from build123d import *

# Parameters (mm, degrees)
ESBO_O1_R             = 5
EXTRUS_O1_DEPTH       = 29
ESBO_O1_3_R           = 6.35
EXTRUS_O2_DEPTH       = 3
ESBO_O2_R             = 1.75
CORTE_EXTRUS_O1_DEPTH = 7.5
CHANFRO1_SIZE         = 0.5


with BuildPart() as part:
    # Esbo_o1 → Extrus_o1 (new body)
    with BuildSketch(Plane.XY):
        with Locations(Location((0, 0, 0), (0, 0, 180))):
            Circle(ESBO_O1_R)
    extrude(amount=EXTRUS_O1_DEPTH)

    # Esbo_o1_3 → Extrus_o2 (add)
    with BuildSketch(Plane.XY):
        Circle(ESBO_O1_3_R)
    extrude(amount=-EXTRUS_O2_DEPTH)

    # Esbo_o2 → Corte-extrus_o1 (cut, symmetric)
    with BuildSketch(Plane(origin=(0, 0, 0), x_dir=(0, 0, -1), z_dir=(1, 0, 0))):
        with Locations(Location((-25.5, 0, 0), (0, 0, 180))):
            Circle(ESBO_O2_R)
    extrude(amount=CORTE_EXTRUS_O1_DEPTH, both=True, mode=Mode.SUBTRACT)

    # Chanfro1
    chanfro1_edges = [part.edges().sort_by_distance(p)[0] for p in [
        (5, 0, 29),
    ]]
    chamfer(chanfro1_edges, length=CHANFRO1_SIZE)


solid = part.part
Geometry check sheet. Reference: the model listing, model coordinates, mm. Round coordinates to 2 decimals unless told otherwise and drop trailing zeros. Loops run counter-clockwise (first coordinate to the right, second up) from the corner with the lowest first, then second, coordinate; pieces in that order, holes last.
Item 1: Mould release check, pull along Y, two halves, no side actions. Record for faces 1 (the cylindrical face through (-4.77, -1.5, 14.05)), 2 (the flat face through (2, -5, 0)), 3 (the cylindrical face through (0.07, -0.08, 23.75)): pulls with the +Y half, pulls with the -Y half, needs draft (parallel to the pull), parting line crosses it, or undercut.
Item 2: Cross-section at D-D on z = 14.5. Record the boundary of the cut face in (x, y), then the cut area to 3 significant figures.
Item 3: Thickness scan on line 1 (Z direction, x = -3.25, y = 4.5); line 2 (Z direction, x = -1.75, y = -1); line 3 (X direction, y = -0.25, z = 5). Record the ranges inside material, lowest first.
Item 4: Cross-section at A-A on y = 0. Record the boundary of the cut face in (x, z).
Item 5: Cross-section at B-B on x = 0. Record the boundary of the cut face in (y, z), then the cut area to 3 significant figures.
Item 6: Gauge pin test, flat ends, axial feed: pin 1 (3 mm diameter, centred on x = -2, z = 14.5, fed in from +Y); pin 2 (1 mm diameter, centred on x = 5, z = 10.5, fed in from +Y); pin 3 (4.5 mm diameter, centred on y = 0, z = 25.5, fed in from -X). Record the tip position at first contact, or that the pin passes through.
Item 7: Cross-section at C-C on z = 25.5. Record the boundary of the cut face in (x, y).
Answer sheet:
1. face 1: parting line crosses it
1. face 2: needs draft
1. face 3: undercut
2. outline: circle Ø10 at (0, 0)
2. area: 78.5 mm2
3. line 1: z = -3 to 0
3. line 2: z = -3 to 24.06, 26.94 to 29
3. line 3: x = -4.99 to 4.99
4. outline: (-6.35, -3) - (6.35, -3) - (6.35, 0) - (5, 0) - (5, 23.75) - (-5, 23.75) - (-5, 0) - (-6.35, 0) - close; (-5, 27.25) - (5, 27.25) - (5, 28.5) - (4.5, 29) - (-4.5, 29) - (-5, 28.5) - close
5. outline: (-6.35, -3) - (6.35, -3) - (6.35, 0) - (5, 0) - (5, 28.5) - (4.5, 29) - (-4.5, 29) - (-5, 28.5) - (-5, 0) - (-6.35, 0) - close; hole circle Ø3.5 at (0, 25.5)
5. area: 318 mm2
6. pin 1: stops at y = 4.97
6. pin 2: stops at y = 2.18
6. pin 3: stops at x = -5
7. outline: (-4.68, -1.75) arc R5 ccw to (4.68, -1.75) - close; (-4.68, 1.75) - (4.68, 1.75) arc R5 ccw to start
